Part model, mm, in its own coordinate system. Face numbers are marked on the shaded views. Give positions to 0.01 mm unless a question says otherwise; leave off trailing zeros. Order: outer loops, then holes, each group sorted by start corner. A loop starts at its lowest first (then second) coordinate and runs counter-clockwise, first axis right, second up.
1. Slice it at A-A on y = 0. List the corners of the cut face in (x, z).
2. Slice it at B-B on z = 1.65. List the corners of the cut face in (x, y) (3 decimals), and give its area (3 significant figures).
3. Slice it at D-D on x = 12. List the corners of the cut face in (y, z).
4. Slice it at C-C on y = -1.75. List the corners of the cut face in (x, z), and give its area (3 significant figures).
5. Probe line 1 (Y direction, x = 0, z = 2.85); line 2 (X direction, y = 0.25, z = 1.7); line 3 (X direction, y = -2.25, z = 0.9). List the from-to ranges inside material, lowest first.
6. Drop a flat-ended pin along its axis: pin 1 Ø1.5 at (x, y) = (1, -1) entering from -Z. Give the stop position or say it passes through.
7. Mould opens along Y. For the marked faces 1, 2 and 3 say: +Y half, -Y half, draft (parallel to the pull), parting line (faces both ways), or undercut.
from build123d import *

# Parameters (mm, degrees)
ESQUISSE1_R             = 2.5
ESQUISSE1_R_2           = 1.5
BOSS_EXTRU_1_DEPTH      = 3
ESQUISSE1_4_R           = 2.5
ESQUISSE1_4_R_2         = 1.5
ENL_V_MAT_EXTRU_1_DEPTH = 2


with BuildPart() as part:
    # Esquisse1 → Boss.-Extru.1 (new body)
    # profile 1 of 2: a face of its own
    with BuildSketch(Plane.XY):
        with BuildLine():
            ThreePointArc((20.15, 2.996247653), (23, 0), (20.15, -2.996247653))
            Line((20.15, -2.996247653), (0.2, -3.994996871))
            ThreePointArc((0.2, -3.994996871), (-4, 0), (0.2, 3.994996871))
            Line((0.2, 3.994996871), (20.15, 2.996247653))
        make_face()
        Circle(ESQUISSE1_R, mode=Mode.SUBTRACT)
        with Locations((20, 0)):
            Circle(ESQUISSE1_R_2, mode=Mode.SUBTRACT)
    # profile 2 of 2: a face of its own
    with BuildSketch(Plane.XY):
        Circle(ESQUISSE1_R)
        Circle(ESQUISSE1_R_2, mode=Mode.SUBTRACT)
    extrude(amount=BOSS_EXTRU_1_DEPTH)

    # Esquisse1_4 → Enl_v. mat.-Extru.1 (cut)
    with BuildSketch(Plane.XY):
        Circle(ESQUISSE1_4_R)
        Circle(ESQUISSE1_4_R_2, mode=Mode.SUBTRACT)
    extrude(amount=ENL_V_MAT_EXTRU_1_DEPTH, mode=Mode.SUBTRACT)


solid = part.part
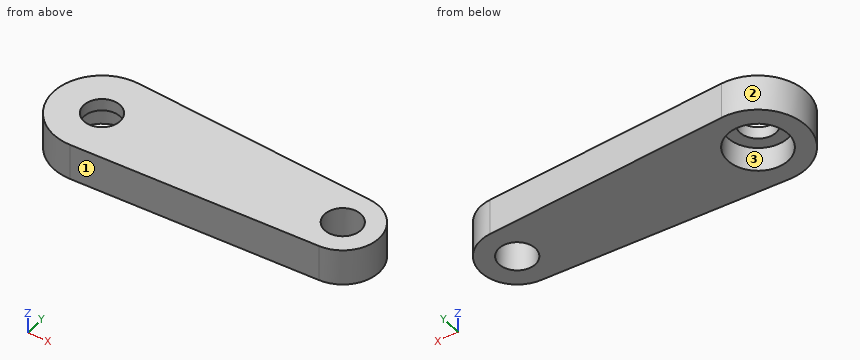
Data:
1. outline: (-4, 0) - (-2.5, 0) - (-2.5, 2) - (-1.5, 2) - (-1.5, 3) - (-4, 3) - close; (1.5, 2) - (2.5, 2) - (2.5, 0) - (18.5, 0) - (18.5, 3) - (1.5, 3) - close; (21.5, 0) - (23, 0) - (23, 3) - (21.5, 3) - close
2. outline: (0.2, -3.995) - (20.15, -2.996) arc R3 ccw to (20.15, 2.996) - (0.2, 3.995) arc R4 ccw (long way) to start; hole circle Ø5 at (0, 0); hole circle Ø3 at (20, 0)
2. area: 153 mm2
3. outline: (-3.4, 0) - (3.4, 0) - (3.4, 3) - (-3.4, 3) - close
4. outline: (-3.6, 0) - (-1.79, 0) - (-1.79, 2) - (1.79, 2) - (1.79, 0) - (22.44, 0) - (22.44, 3) - (-3.6, 3) - close
4. area: 71.0 mm2
5. line 1: y = -4 to -1.5, 1.5 to 4
5. line 2: x = -3.99 to -2.49, 2.49 to 18.52, 21.48 to 22.99
5. line 3: x = -3.31 to -1.09, 1.09 to 21.98
6. pin 1: stops at z = 2
7. face 1: -Y half
7. face 2: parting line
7. face 3: undercut
